Model file for the job. Use its own axes, mm. Face numbers are marked on the shaded views. A direction names the side the tool comes from. Round coordinates to 2 decimals unless told otherwise and drop trailing zeros. Order: outer loops, then holes, each group sorted by start corner. A loop starts at its lowest first (then second) coordinate and runs counter-clockwise, first axis right, second up. Notation, with made-up numbers: M 44.25,-23.5 L 54.25,-23.5 A32 cw 54.25,10.5 Z; hole C 60,61.25 d1. An arc over 180 degrees is marked long. Return JSON: item names as keys, results as strings. Group by question number.
Item 1: Pull direction X, two halves, no side cores. Call the marked faces 1, 2, 3 and 4: pulls with the +X half, pulls with the -X half, needs draft (parallel to the pull), parting line crosses it, or undercut.
Item 2: Slice it at D-D on x = 141.5. Write the cut outline in (y, z).
Item 3: Which spindle directions (+Z, -Z, +X, -X, +Y, -Y) get a long thin tool onto all of the face, cutting with end or side? Do the marked faces 5 and 6. Say none if no direction does.
Item 4: Slice it at C-C on z = -69.5. Write the cut outline in (x, y).
Item 5: Probe line 1 along Y through (x, z) = (170.25, -39.5); line 2 along Z through (x, y) = (41, 25.5); line 3 along Z through (x, y) = (88, 7). List the from-to ranges inside material, lowest first.
Item 6: Pin check, flat tips, straight feed: pin 1 Ø4 at (x, z) = (61.5, -37.5) entering from +Y; pin 2 Ø1.6 at (x, y) = (11, 24) entering from +Z; pin 3 Ø12 at (x, z) = (30, -53) entering from +Y; pin 4 Ø0.6 at (x, y) = (13.5, 3.5) entering from +Z. Stop position of each tip, or through.
Item 7: Slice it at B-B on x = 31. Write the cut outline in (y, z).
from build123d import *

# Parameters (mm, degrees)
EXTRUDE_1_DEPTH             = 28
SKETCH_3_W                  = 8
SKETCH_3_H                  = 106
EXTRUDE_2_DEPTH             = 3
EXTRUDE_2_2_DEPTH           = 3
EXTRUDE_START               = -3
EXTRUDE_3_DEPTH             = 3
HOLE_WIZARD_M51_D           = 2
HOLE_WIZARD_M51_CBORE_D     = 3
HOLE_WIZARD_M51_CBORE_DEPTH = 1
SKETCH_17_W                 = 56
SKETCH_17_H                 = 22
SKETCH_17_W_2               = 7
SKETCH_17_H_2               = 7
CUT_EXTRUDE_2_DEPTH         = 1.5
CUT_EXTRUDE_3_REACH         = 208.345
SKETCH_18_W                 = 51
SKETCH_18_H                 = 16
SKETCH_19_W                 = 8
SKETCH_19_H                 = 8
EXTRUDE_4_DEPTH             = 2
HOLE_WIZARD_3_0_3_1_D       = 3
HOLE_WIZARD_3_0_3_1_DEPTH   = 5
HOLE_WIZARD_3_0_3_1_TIP     = 0.901290929
HOLE_WIZARD_2_0_2_1_D       = 2
HOLE_WIZARD_2_0_2_1_DEPTH   = 5
HOLE_WIZARD_2_0_2_1_TIP     = 0.600860619
CUT_EXTRUDE_4_DEPTH         = 1.5
FILLET_1_R                  = 3
SKETCH_28_W                 = 5
SKETCH_28_H                 = 106
EXTRUDE_5_DEPTH             = 3
SKETCH_29_W                 = 22
SKETCH_29_H                 = 22
CUT_EXTRUDE_5_DEPTH         = 1.5
SKETCH_30_R                 = 7
CUT_EXTRUDE_6_DEPTH         = 1.5
HOLE_WIZARD_2_0_2_2_D       = 2
HOLE_WIZARD_2_0_2_2_DEPTH   = 1.5
HOLE_WIZARD_2_0_2_2_TIP     = 0.600860619


with BuildPart() as part:
    # Sketch 1 → Extrude 1 (new body)
    with BuildSketch(Plane(origin=(0, 0, 0), x_dir=(1, 0, 0), z_dir=(0, 1, 0))):
        with BuildLine():
            Line((8, 0), (164, 0))
            ThreePointArc((164, 0), (169.656854249, 2.343145751), (172, 8))
            Line((172, 8), (172, 104))
            ThreePointArc((172, 104), (169.656854249, 109.656854249), (164, 112))
            Line((164, 112), (8, 112))
            ThreePointArc((8, 112), (2.343145751, 109.656854249), (0, 104))
            Line((0, 104), (0, 8))
            ThreePointArc((0, 8), (2.343145751, 2.343145751), (8, 0))
        make_face()
        with BuildLine():
            Line((8, 109), (164, 109))
            ThreePointArc((164, 109), (167.535533906, 107.535533906), (169, 104))
            Line((169, 104), (169, 8))
            ThreePointArc((169, 8), (167.535533906, 4.464466094), (164, 3))
            Line((164, 3), (8, 3))
            ThreePointArc((8, 3), (4.464466094, 4.464466094), (3, 8))
            Line((3, 8), (3, 104))
            ThreePointArc((3, 104), (4.464466094, 107.535533906), (8, 109))
        make_face(mode=Mode.SUBTRACT)
    extrude(amount=EXTRUDE_1_DEPTH)



with BuildPart() as body_2:
    # Sketch 3 → Extrude 2 (new body)
    with BuildSketch(Plane(origin=(0, 0, 0), x_dir=(1, 0, 0), z_dir=(0, 1, 0))):
        with Locations((13, 56)):
            Rectangle(SKETCH_3_W, SKETCH_3_H)
    extrude(amount=EXTRUDE_2_DEPTH)


with BuildPart() as body_3:
    # Sketch 3 → Extrude 2 2 (new body)
    with BuildSketch(Plane(origin=(0, 0, 0), x_dir=(1, 0, 0), z_dir=(0, 1, 0))):
        with Locations((62, 56)):
            Rectangle(SKETCH_3_W, SKETCH_3_H)
    extrude(amount=EXTRUDE_2_2_DEPTH)


with BuildPart() as part_1:
    add(part.part)

    add(body_2.part)  # Extrude 3 merges body 2

    add(body_3.part)  # Extrude 3 merges body 3
    # Sketch 6 → Extrude 3 (add)
    with BuildSketch(Plane(origin=(0, 0, 0), x_dir=(1, 0, 0), z_dir=(0, 1, 0)).offset(EXTRUDE_START)):
        with BuildLine():
            Line((0, 8), (0, 104))
            ThreePointArc((0, 104), (2.343145751, 109.656854249), (8, 112))
            Line((8, 112), (164, 112))
            ThreePointArc((164, 112), (169.656854249, 109.656854249), (172, 104))
            Line((172, 104), (172, 8))
            ThreePointArc((172, 8), (169.656854249, 2.343145751), (164, 0))
            Line((164, 0), (8, 0))
            ThreePointArc((8, 0), (2.343145751, 2.343145751), (0, 8))
        make_face()
    extrude(amount=EXTRUDE_3_DEPTH)

    # Hole Wizard M51 (through all)
    with Locations(Plane(origin=(0, -3, 0), x_dir=(-1, 0, 0), z_dir=(0, -1, 0))):
        with Locations((-6, 6), (-6, 106), (-166, 106), (-166, 6), (-86, 5), (-86, 107)):
            CounterBoreHole(HOLE_WIZARD_M51_D / 2, HOLE_WIZARD_M51_CBORE_D / 2, HOLE_WIZARD_M51_CBORE_DEPTH)

    # Sketch 17 → Cut-Extrude 2 (cut)
    with BuildSketch(Plane.XY):
        with Locations((37, 15)):
            Rectangle(SKETCH_17_W, SKETCH_17_H)
        with Locations((37, 0.5)):
            Rectangle(SKETCH_17_W_2, SKETCH_17_H_2)
    extrude(amount=-CUT_EXTRUDE_2_DEPTH, mode=Mode.SUBTRACT)

    # Sketch 18 → Cut-Extrude 3 (cut, up to next)
    with BuildSketch(Plane.XY.offset(-1.5), mode=Mode.PRIVATE) as cut_extrude_3_sk1:
        with Locations((37, 14)):
            Rectangle(SKETCH_18_W, SKETCH_18_H)
    cut_extrude_3_tool1 = extrude(cut_extrude_3_sk1.sketch, amount=-CUT_EXTRUDE_3_REACH, mode=Mode.PRIVATE) & part_1.part
    add(cut_extrude_3_tool1.solids().sort_by_distance((37, 14, -1.5))[0], mode=Mode.SUBTRACT)

    # Sketch 19 → Extrude 4 (add)
    with BuildSketch(Plane(origin=(0, 3, 0), x_dir=(1, 0, 0), z_dir=(0, 1, 0))):
        with Locations((13, 95)):
            Rectangle(SKETCH_19_W, SKETCH_19_H)
        with Locations((62, 95)):
            Rectangle(SKETCH_19_W, SKETCH_19_H)
        with Locations((13, 37)):
            Rectangle(SKETCH_19_W, SKETCH_19_H)
        with Locations((62, 37)):
            Rectangle(SKETCH_19_W, SKETCH_19_H)
    extrude(amount=EXTRUDE_4_DEPTH)

    # Hole Wizard 3.0 _3_1
    with Locations(Plane(origin=(0, 5, 0), x_dir=(1, 0, 0), z_dir=(0, 1, 0))):
        with Locations((13, 95), (62, 95), (62, 37), (13, 37)):
            Hole(HOLE_WIZARD_3_0_3_1_D / 2, depth=HOLE_WIZARD_3_0_3_1_DEPTH)
            with Locations((0, 0, -(HOLE_WIZARD_3_0_3_1_DEPTH + HOLE_WIZARD_3_0_3_1_TIP / 2))):  # 118° drill point
                Cone(0, HOLE_WIZARD_3_0_3_1_D / 2, HOLE_WIZARD_3_0_3_1_TIP, mode=Mode.SUBTRACT)

    # Hole Wizard 2.0 _2_1
    with Locations(Plane.XY.offset(-1.5)):
        with Locations((37, 1), (11, 24), (63, 24)):
            Hole(HOLE_WIZARD_2_0_2_1_D / 2, depth=HOLE_WIZARD_2_0_2_1_DEPTH)
            with Locations((0, 0, -(HOLE_WIZARD_2_0_2_1_DEPTH + HOLE_WIZARD_2_0_2_1_TIP / 2))):  # 118° drill point
                Cone(0, HOLE_WIZARD_2_0_2_1_D / 2, HOLE_WIZARD_2_0_2_1_TIP, mode=Mode.SUBTRACT)

    # Sketch 27 → Cut-Extrude 4 (cut)
    with BuildSketch(Plane(origin=(0, 28, 0), x_dir=(1, 0, 0), z_dir=(0, 1, 0))):
        with BuildLine():
            Line((170.5, 8), (170.5, 104))
            ThreePointArc((170.5, 104), (168.596194078, 108.596194078), (164, 110.5))
            Line((164, 110.5), (8, 110.5))
            ThreePointArc((8, 110.5), (3.403805922, 108.596194078), (1.5, 104))
            Line((1.5, 104), (1.5, 8))
            ThreePointArc((1.5, 8), (3.403805922, 3.403805922), (8, 1.5))
            Line((8, 1.5), (164, 1.5))
            ThreePointArc((164, 1.5), (168.596194078, 3.403805922), (170.5, 8))
        make_face()
    extrude(amount=-CUT_EXTRUDE_4_DEPTH, mode=Mode.SUBTRACT)

    # Fillet 1
    fillet_1_edges = [part_1.edges().sort_by_distance(p)[0] for p in [
        (11.5, 6, -2.25),
        (11.5, 22, -2.25),
        (62.5, 22, -2.25),
        (62.5, 6, -2.25),
    ]]
    fillet(fillet_1_edges, radius=FILLET_1_R)

    # Sketch 28 → Extrude 5 (add)
    with BuildSketch(Plane(origin=(0, 0, 0), x_dir=(1, 0, 0), z_dir=(0, 1, 0))):
        with Locations((106.5, 56)):
            Rectangle(SKETCH_28_W, SKETCH_28_H)
        with Locations((136.5, 56)):
            Rectangle(SKETCH_28_W, SKETCH_28_H)
    extrude(amount=EXTRUDE_5_DEPTH)

    # Sketch 29 → Cut-Extrude 5 (cut)
    with BuildSketch(Plane(origin=(172, 0, 0), x_dir=(0, 0, -1), z_dir=(1, 0, 0))):
        with Locations((31, 13)):
            Rectangle(SKETCH_29_W, SKETCH_29_H)
    extrude(amount=-CUT_EXTRUDE_5_DEPTH, mode=Mode.SUBTRACT)

    # Sketch 30 → Cut-Extrude 6 (cut)
    with BuildSketch(Plane(origin=(170.5, 0, 0), x_dir=(0, 0, -1), z_dir=(1, 0, 0))):
        with Locations((31, 13)):
            Circle(SKETCH_30_R)
    extrude(amount=-CUT_EXTRUDE_6_DEPTH, mode=Mode.SUBTRACT)

    # Hole Wizard 2.0 _2_2
    with Locations(Plane(origin=(170.5, 0, 0), x_dir=(0, 0, -1), z_dir=(1, 0, 0))):
        with Locations((22.5, 21.5), (39.5, 21.5), (39.5, 4.5), (22.5, 4.5)):
            Hole(HOLE_WIZARD_2_0_2_2_D / 2, depth=HOLE_WIZARD_2_0_2_2_DEPTH)
            with Locations((0, 0, -(HOLE_WIZARD_2_0_2_2_DEPTH + HOLE_WIZARD_2_0_2_2_TIP / 2))):  # 118° drill point
                Cone(0, HOLE_WIZARD_2_0_2_2_D / 2, HOLE_WIZARD_2_0_2_2_TIP, mode=Mode.SUBTRACT)


solid = part_1.part
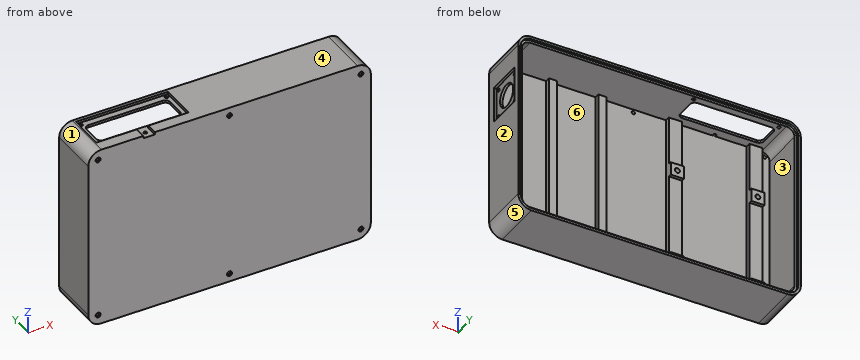
Output values:
{
 "1": {"face 1": "pulls with the -X half", "face 2": "pulls with the +X half", "face 3": "undercut", "face 4": "needs draft"},
 "2": {"outline": "M -3,-112 L 28,-112 L 28,-110.5 L 26.5,-110.5 L 26.5,-109 L 0,-109 L 0,-3 L 26.5,-3 L 26.5,-1.5 L 28,-1.5 L 28,0 L -3,0 Z"},
 "3": {"face 5": "-Z, +X, +Y, -Y", "face 6": "+Y"},
 "4": {"outline": "M 0,-3 L 172,-3 L 172,28 L 170.5,28 L 170.5,26.5 L 169,26.5 L 169,0 L 139,0 L 139,3 L 134,3 L 134,0 L 109,0 L 109,3 L 104,3 L 104,0 L 66,0 L 66,3 L 58,3 L 58,0 L 17,0 L 17,3 L 9,3 L 9,0 L 3,0 L 3,26.5 L 1.5,26.5 L 1.5,28 L 0,28 Z"},
 "5": {"line 1": "-3 to 3.5, 5.5 to 20.5, 22.5 to 26.5", "line 2": "-112 to -109, -3 to -1.5", "line 3": "-112 to -109, -3 to 0"},
 "6": {"pin 1": "y = 5", "pin 2": "z = -109", "pin 3": "y = 0", "pin 4": "z = 0"},
 "7": {"outline": "M -3,-112 L 28,-112 L 28,-110.5 L 26.5,-110.5 L 26.5,-109 L 0,-109 L 0,-3 L 6,-3 L 6,-1.5 L 4,-1.5 L 4,0 L -3,0 Z; M 22,-3 L 26.5,-3 L 26.5,-1.5 L 28,-1.5 L 28,0 L 26,0 L 26,-1.5 L 22,-1.5 Z"}
}
